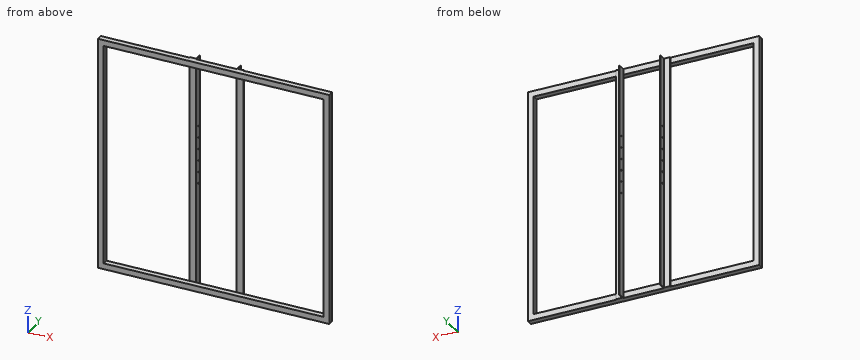
from build123d import *

# Parameters (mm, degrees)
SKETCH1_W           = 800
SKETCH1_H           = 800
SKETCH1_W_2         = 760
SKETCH1_H_2         = 760
BOSS_EXTRUDE1_DEPTH = 20
SKETCH2_W           = 2
SKETCH2_H           = 800
BOSS_EXTRUDE2_DEPTH = 25.3
SKETCH3_R           = 2.1
CUT_EXTRUDE2_DEPTH  = 158
SKETCH4_W           = 21.3
SKETCH4_H           = 800
BOSS_EXTRUDE3_DEPTH = 3.09


with BuildPart() as part:
    # Sketch1 → Boss-Extrude1 (new body)
    with BuildSketch(Plane(origin=(0, 0, 0), x_dir=(1, 0, 0), z_dir=(0, 1, 0))):
        Rectangle(SKETCH1_W, SKETCH1_H)
        Rectangle(SKETCH1_W_2, SKETCH1_H_2, mode=Mode.SUBTRACT)
    extrude(amount=BOSS_EXTRUDE1_DEPTH)

    # Sketch2 → Boss-Extrude2 (add)
    with BuildSketch(Plane(origin=(0, 20, 0), x_dir=(1, 0, 0), z_dir=(0, 1, 0))):
        with Locations((-71, 0)):
            Rectangle(SKETCH2_W, SKETCH2_H)
        with Locations((71, 0)):
            Rectangle(SKETCH2_W, SKETCH2_H)
    extrude(amount=BOSS_EXTRUDE2_DEPTH)

    # Sketch3 → Cut-Extrude2 (cut)
    with BuildSketch(Plane.ZY.offset(72)):
        with Locations((0, 32.65)):
            Circle(SKETCH3_R)
        with Locations((-40, 32.65)):
            Circle(SKETCH3_R)
        with Locations((40, 32.65)):
            Circle(SKETCH3_R)
        with Locations((80, 32.65)):
            Circle(SKETCH3_R)
        with Locations((120, 32.65)):
            Circle(SKETCH3_R)
        with Locations((160, 32.65)):
            Circle(SKETCH3_R)
    extrude(amount=-CUT_EXTRUDE2_DEPTH, mode=Mode.SUBTRACT)

    # Sketch4 → Boss-Extrude3 (add)
    with BuildSketch(Plane(origin=(0, 20, 0), x_dir=(1, 0, 0), z_dir=(0, 1, 0))):
        with Locations((82.65, 0)):
            Rectangle(SKETCH4_W, SKETCH4_H)
        with Locations((-82.65, 0)):
            Rectangle(SKETCH4_W, SKETCH4_H)
    extrude(amount=BOSS_EXTRUDE3_DEPTH)


solid = part.part
CAD build for the part. Positions are in the model's coordinates, mm. Round coordinates to 2 decimals unless told otherwise and drop trailing zeros. Write each loop counter-clockwise with the first axis right and the second up, starting at its lowest first coordinate (ties: lowest second). Pieces come first, ordered by that corner, then holes. Notation, with made-up numbers: M 0,3.5 L 48,3.5 A14 cw 48,23.5 Z; hole C -20.75,54.25 d5. An arc over 180 degrees is marked long. Put each result on its own line as item: value. Start each with the question number.
1) Drill centre lines: probe 1 along X at (y, z) = (42.5, 41); probe 2 along Y at (x, z) = (-71.35, 0); probe 3 along X at (y, z) = (5, 318.5). Where is each one in solid material? Low to high. Write a range as [from, to].
2) Saw through at A-A, the plane z = -186. Write the cut outline in (x, y).
3) Pin check, flat tips, straight feed: pin 1 Ø2.5 at (y, z) = (22, -64.5) entering from -X; pin 2 Ø12.5 at (y, z) = (32.5, 175) entering from -X; pin 3 Ø11 at (y, z) = (37, -94) entering from +X. Stop position of each tip, or through.
4) Saw through at B-B, the plane x = -256. Write the cut outline in (y, z).
Resolved:
1. probe 1: [-72, -70], [70, 72]
1. probe 2: [20, 30.55], [34.75, 45.3]
1. probe 3: [-400, -380], [380, 400]
2. outline: M -400,0 L -380,0 L -380,20 L -400,20 Z; M -93.3,20 L -70,20 L -70,45.3 L -72,45.3 L -72,23.09 L -93.3,23.09 Z; M 70,20 L 93.3,20 L 93.3,23.09 L 72,23.09 L 72,45.3 L 70,45.3 Z; M 380,0 L 400,0 L 400,20 L 380,20 Z
3. pin 1: x = -93.3
3. pin 2: x = -72
3. pin 3: x = 72
4. outline: M 0,-400 L 20,-400 L 20,-380 L 0,-380 Z; M 0,380 L 20,380 L 20,400 L 0,400 Z
